Can you work these out from the drawing? Everything is in mm from the part's minimum corner. Give positions to 0.01 mm unless a question says otherwise; leave off trailing zeros. Order: outer loops, then holes, each group sorted by start corner. A loop starts at its lowest first (then second) coordinate and runs counter-clockwise, first axis right, second up. Notation, with made-up numbers: (70, 30) - (86, 30) arc R21 ccw to (86, 51) - close; hole circle Ø11 at (79.5, 38). An arc over 180 degrees is marked (long way). One line per question, with ' | ' between items.
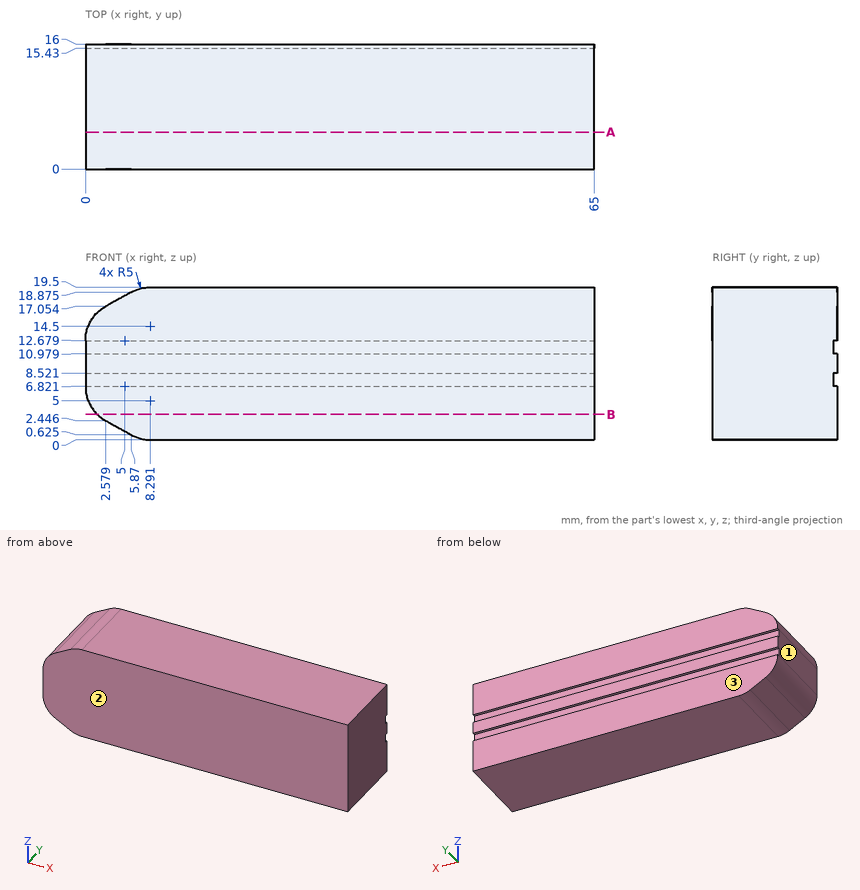
1) Please list where these lines run through material, in increasing order: L1, parallel to Y at x = 13, z = 11.75; L2, parallel to X at y = 5.75, z = 14.75; L3, parallel to X at y = 1, z = 1.25.
Model answer:
L1: y = 0 to 15.43 | L2: x = 0.45 to 65 | L3: x = 4.74 to 65
2) I want a section at A-A (y = 4.75). List the corners of the cut face in (x, z) for me (1 decimal).
Model answer:
outline: (0, 6.8) arc R5 ccw to (2.6, 2.4) - (5.9, 0.6) arc R5 ccw to (8.3, 0) - (65, 0) - (65, 19.5) - (8.3, 19.5) arc R5 ccw to (5.9, 18.9) - (2.6, 17.1) arc R5 ccw to (0, 12.7) - close
3) Thinking about a two-plate mould opening in Y: for the marked faces 1, 2 and 3, which applies, +Y half, -Y half, draft (parallel to the pull), parting line (faces both ways), or undercut?
Model answer:
face 1: draft | face 2: -Y half | face 3: +Y half
4) I want a section at B-B (z = 3.25). List the corners of the cut face in (x, y) for me.
Model answer:
outline: (1.5, 0) - (65, 0) - (65, 16) - (1.5, 16) - close
5) I'm going to push a flat-ended pin straight in: P1, Ø0.5, axis at x = 46, z = 7.5, coming from the +Y side. Where does the tip first touch, or does it pass through?
Model answer:
P1: stops at y = 15.43
